Build history of the part. All positions in model axes, mm. Face numbers are marked on the shaded views. A direction names the side the tool comes from. Round coordinates to 2 decimals unless told otherwise and drop trailing zeros. Loops run counter-clockwise (first coordinate to the right, second up) from the corner with the lowest first, then second, coordinate; pieces in that order, holes last. Notation, with made-up numbers: (-14, 57) -> (7, 57) arc R19 ccw to (7, 89) -> close; hole circle Ø7 at (16.25, 3.25). An arc over 180 degrees is marked (long way). Put each result on its own line as item: value. Start each with the question number.
Item 1: Cut at D-D, the plane z = 142. List the corners of the cut face in (x, y), plus the area to 3 significant figures.
Item 2: Flat gauge pins, fed straight in: pin 1 Ø5 at (y, z) = (-620, 163.5) entering from -X; pin 2 Ø24 at (x, z) = (190.5, 189) entering from +Y. Where does each tip first touch, or does it go through?
Item 3: Cut at A-A, the plane x = -478. List the corners of the cut face in (y, z).
Item 4: Cut at B-B, the plane y = -450. List the corners of the cut face in (x, z), plus the area to 3 significant figures.
Item 5: Pull direction Z, two halves, no side cores. Call the marked faces 1, 2, 3 and 4: +Z half, -Z half, draft (parallel to the pull), parting line (faces both ways), or undercut.
Item 6: Cut at C-C, the plane x = 116. List the corners of the cut face in (y, z).
Item 7: Tool access for the marked faces 5, 6, 7, 8 and 9: list every direction of +Z, -Z, +X, -X, +Y, -Y with a clear straight run to the whole face (end or side of a thin tool).
Item 8: Drill centre lines: probe 1 along Y at (x, z) = (537, 187.5); probe 2 along Y at (x, z) = (-524, -224.5); probe 3 along Z at (x, y) = (589, -220). Where is each one in solid material? Low to high. Write a range as [from, to].
```python
from build123d import *

# Parameters (mm, degrees)
F1_DEPTH = 700
F3_DEPTH = 1300.001
F4_W     = 200
F4_H     = 300
F5_DEPTH = 300.001


with BuildPart() as f1:
    # F0 (on Front) → F1 (new body)
    with BuildSketch(Plane.XZ):
        Polygon((650, -350), (650, 350), (150, 350), (-250, -50), (-650, -50), (-650, -350), align=None)
    extrude(amount=F1_DEPTH)

    # F2 (on face) → F3 (cut, through all)
    with BuildSketch(Plane.YZ.offset(650)):
        with BuildLine():
            ThreePointArc((-550, 170.143622), (-535.355339, 134.788283), (-500, 120.143622))
            Line((-500, 120.143622), (-200, 120.143622))
            ThreePointArc((-200, 120.143622), (-164.644661, 134.788283), (-150, 170.143622))
            Line((-150, 170.143622), (-150, 200))
            ThreePointArc((-150, 200), (-164.644661, 235.355339), (-200, 250))
            Line((-200, 250), (-500, 250))
            ThreePointArc((-500, 250), (-535.355339, 235.355339), (-550, 200))
            Line((-550, 200), (-550, 170.143622))
        make_face()
    extrude(amount=-F3_DEPTH, mode=Mode.SUBTRACT)

    # F4 (on face) → F5 (cut, through all)
    with BuildSketch(Plane.XY.offset(-50)):
        with Locations((-550, -350)):
            Rectangle(F4_W, F4_H)
    extrude(amount=-F5_DEPTH, mode=Mode.SUBTRACT)


solid = f1.part
```
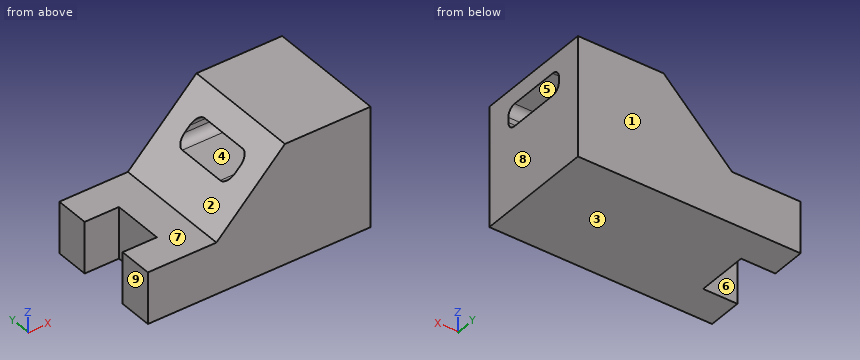
Reply:
1. outline: (-58, -700) -> (650, -700) -> (650, -541.33) -> (-58, -541.33) -> close; (-58, -158.67) -> (650, -158.67) -> (650, 0) -> (-58, 0) -> close
1. area: 225,000 mm^2
2. pin 1: stops at x = -39
2. pin 2: stops at y = 0
3. outline: (-700, -350) -> (-500, -350) -> (-500, -50) -> (-700, -50) -> close; (-200, -350) -> (0, -350) -> (0, -50) -> (-200, -50) -> close
4. outline: (-450, -350) -> (650, -350) -> (650, 120.14) -> (-79.86, 120.14) -> (-250, -50) -> (-450, -50) -> close; (50, 250) -> (650, 250) -> (650, 350) -> (150, 350) -> close
4. area: 524,000 mm^2
5. face 1: draft
5. face 2: +Z half
5. face 3: -Z half
5. face 4: undercut
6. outline: (-700, -350) -> (0, -350) -> (0, 316) -> (-700, 316) -> close; hole (-550, 170.14) arc R50 ccw to (-500, 120.14) -> (-200, 120.14) arc R50 ccw to (-150, 170.14) -> (-150, 200) arc R50 ccw to (-200, 250) -> (-500, 250) arc R50 ccw to (-550, 200) -> close
7. face 5: +X, -X
7. face 6: +Z, -Z, -X
7. face 7: +Z, -X, +Y, -Y
7. face 8: +Z, -Z, +X, +Y, -Y
7. face 9: +Z, -Z, -X, +Y, -Y
8. probe 1: y = [-700, -550], [-150, 0]
8. probe 2: y = [-700, -500], [-200, 0]
8. probe 3: z = [-350, 120.14], [250, 350]
